from build123d import *

# Parameters (mm, degrees)
SKETCH1_R           = 16
BOSS_EXTRUDE1_DEPTH = 41.9
SKETCH2_R           = 1.5
CUT_EXTRUDE1_DEPTH  = 5
BOSS_EXTRUDE2_DEPTH = 3
SKETCH4_R           = 3
BOSS_EXTRUDE3_DEPTH = 16.25
SKETCH5_R           = 18.5
BOSS_EXTRUDE4_DEPTH = 68.1


with BuildPart() as part:
    # Sketch1 → Boss-Extrude1 (new body)
    with BuildSketch(Plane.XY):
        Circle(SKETCH1_R)
    extrude(amount=BOSS_EXTRUDE1_DEPTH)

    # Sketch2 → Cut-Extrude1 (cut)
    with BuildSketch(Plane.XY.offset(41.9)):
        with Locations((-9.192388155, 9.192388155)):
            Circle(SKETCH2_R)
        with Locations((9.192388155, 9.192388155)):
            Circle(SKETCH2_R)
        with Locations((9.192388155, -9.192388155)):
            Circle(SKETCH2_R)
        with Locations((-9.192388155, -9.192388155)):
            Circle(SKETCH2_R)
    extrude(amount=-CUT_EXTRUDE1_DEPTH, mode=Mode.SUBTRACT)

    # Sketch3 → Boss-Extrude2 (add)
    with BuildSketch(Plane.XY.offset(41.9)):
        with BuildLine():
            Line((9, 4.358898944), (9, -4.358898944))
            ThreePointArc((9, -4.358898944), (0, -10), (-9, -4.358898944))
            Line((-9, -4.358898944), (-9, 4.358898944))
            ThreePointArc((-9, 4.358898944), (0, 10), (9, 4.358898944))
        make_face()
    extrude(amount=BOSS_EXTRUDE2_DEPTH)

    # Sketch4 → Boss-Extrude3 (add)
    with BuildSketch(Plane.XY.offset(44.9)):
        Circle(SKETCH4_R)
    extrude(amount=BOSS_EXTRUDE3_DEPTH)

    # Sketch5 → Boss-Extrude4 (add)
    with BuildSketch(Plane(origin=(0, 0, 0), x_dir=(-1, 0, 0), z_dir=(0, 0, -1))):
        Circle(SKETCH5_R)
    extrude(amount=BOSS_EXTRUDE4_DEPTH)


solid = part.part
Verification items for the finished model (mm, model axes). A direction names the side the tool comes from. Round coordinates to 2 decimals unless told otherwise and drop trailing zeros. Loops run counter-clockwise (first coordinate to the right, second up) from the corner with the lowest first, then second, coordinate; pieces in that order, holes last. Notation, with made-up numbers: (14, 1.5) - (35, 1.5) arc R23 cw to (35, 35.5) - close; hole circle Ø6 at (82.5, -35). An arc over 180 degrees is marked (long way). Write item = value, one per line.
Q1. Sectioned sample at D-D on y = -13. Record the boundary of the cut face in (x, z).
Here are the results:
outline = (-13.16, -68.1) - (13.16, -68.1) - (13.16, 0) - (9.33, 0) - (9.33, 41.9) - (-9.33, 41.9) - (-9.33, 0) - (-13.16, 0) - close
Q2. Depth check by flat-ended pin: pin 1 (2.5 mm diameter, centred on y = -1.5, z = 43, fed in from -X); pin 2 (1.5 mm diameter, centred on y = 0, z = 43, fed in from +X); pin 3 (2.5 mm diameter, centred on x = -9.5, y = 9, fed in from +Z); pin 4 (9 mm diameter, centred on x = -4, y = 0.5, fed in from +Z). Enter the tip coordinate at first touch or a pass-through.
Here are the results:
pin_1 = -15.97
pin_2 = 9
pin_3 = 41.9
pin_4 = 61.15
Q3. Tool access check on faces 1 (the cylindrical face through (0, 10, 43)), 2 (the flat face through (9, 0, 43)), 3 (the flat face through (-9, 9, 36.9)). Record the directions out of +Z, -Z, +X, -X, +Y, -Y that give a thin tool (end or side, any length) a straight path to the whole face; none if there is none.
Here are the results:
face_1 = +Z, +Y
face_2 = +Z, +X, +Y, -Y
face_3 = +Z
Q4. Sectioned sample at A-A on x = 0. Record the boundary of the cut face in (y, z).
Here are the results:
outline = (-18.5, -68.1) - (18.5, -68.1) - (18.5, 0) - (16, 0) - (16, 41.9) - (10, 41.9) - (10, 44.9) - (3, 44.9) - (3, 61.15) - (-3, 61.15) - (-3, 44.9) - (-10, 44.9) - (-10, 41.9) - (-16, 41.9) - (-16, 0) - (-18.5, 0) - close
Q5. Mould release check, pull along X, two halves, no side actions. Record for faces 4 (the flat face through (-9, 0, 43)), 5 (the flat face through (9, -9, 36.9)), 6 (the flat face through (0, 0, -68.1)): +X half, -X half, draft (parallel to the pull), parting line (faces both ways), or undercut.
Here are the results:
face_4 = -X half
face_5 = undercut
face_6 = draft
Q6. Sectioned sample at B-B on y = 0. Record the boundary of the cut face in (x, z).
Here are the results:
outline = (-18.5, -68.1) - (18.5, -68.1) - (18.5, 0) - (16, 0) - (16, 41.9) - (9, 41.9) - (9, 44.9) - (3, 44.9) - (3, 61.15) - (-3, 61.15) - (-3, 44.9) - (-9, 44.9) - (-9, 41.9) - (-16, 41.9) - (-16, 0) - (-18.5, 0) - close
Q7. Material ranges on L1, parallel to Z at x = 8.5, y = -6.5; L2, parallel to Z at x = -14.5, y = 11; L3, parallel to Y at x = 0, z = 32, recorded low to high.
Here are the results:
L1 = -68.1 to 41.9
L2 = -68.1 to 0
L3 = -16 to 16
Q8. Sectioned sample at C-C on z = -27. Record the boundary of the cut face in (x, y), plus the area to 3 significant figures.
Here are the results:
outline = circle Ø37 at (0, 0)
area = 1,080 mm^2
